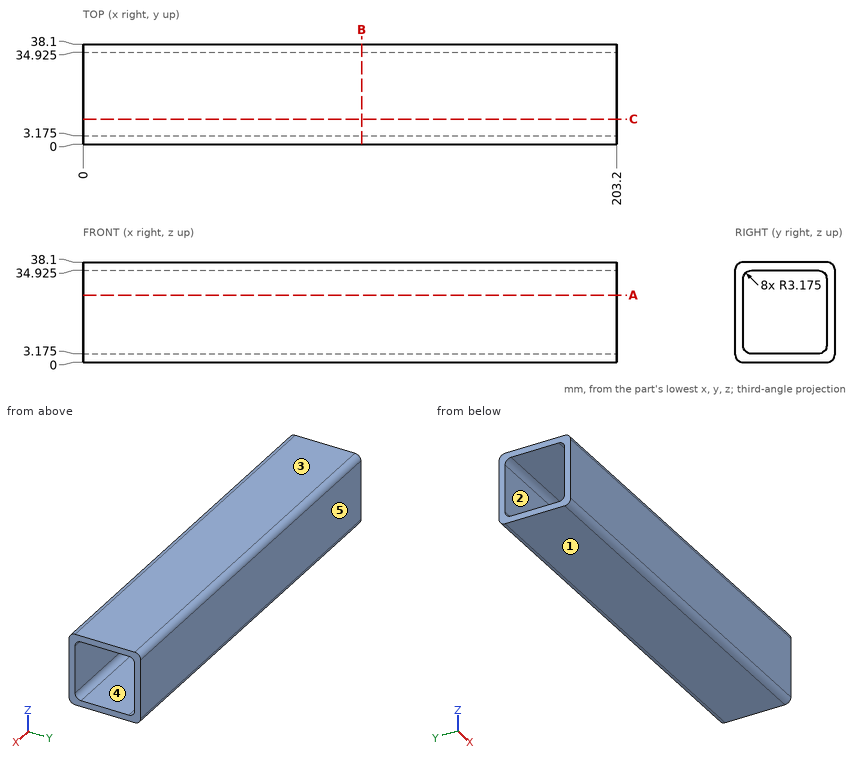
Source: three-view drawing plus pictorial views. Frame: mm from the lowest corner of the part. A direction names the side the tool comes from. Round coordinates to 2 decimals unless told otherwise and drop trailing zeros. Write each loop counter-clockwise with the first axis right and the second up, starting at its lowest first coordinate (ties: lowest second). Pieces come first, ordered by that corner, then holes. Notation, with made-up numbers: M 69,19.5 L 99,19.5 A15 ccw 99,42.5 Z; hole C -27,22.25 d6. An arc over 180 degrees is marked long. Write item = value, one per line.
Item 1: Material intervals for line 1 along Y through (x, z) = (79, 18) (3 decimals); line 2 along Y through (x, z) = (167, 5), sorted ascending. Write a range as [from, to].
Findings:
line_1 = [0, 3.175], [34.925, 38.1]
line_2 = [0, 3.48], [34.62, 38.1]
Item 2: Pin query (flat end, axial travel): P1, Ø4, axis at y = 32.5, z = 28, coming from the +X side. Return the tip coordinate at first contact, or that it passes through.
Findings:
P1 = through
Item 3: Section query A-A on z = 25.5. Return loops of the section in (x, y) (3 decimals), then the cut area to 3 significant figures.
Findings:
outline = M 0,0 L 203.2,0 L 203.2,3.175 L 0,3.175 Z; M 0,34.925 L 203.2,34.925 L 203.2,38.1 L 0,38.1 Z
area = 1,290 mm^2
Item 4: Access query for the marked faces 1 and 2. Directions: +Z, -Z, +X, -X, +Y, -Y. A direction counts if a zero-diameter tool reaches every point of the face in a straight line with its end or side. Return the directions, or none.
Findings:
face_1 = -Z, +X, -X, +Y, -Y
face_2 = +X, -X
Item 5: Pull-direction query (Y, two-part tool) for the marked faces 3, 4 and 5; classes: pulls with the +Y half, pulls with the -Y half, needs draft (parallel to the pull), parting line crosses it, or undercut.
Findings:
face_3 = needs draft
face_4 = undercut
face_5 = pulls with the +Y half
Item 6: Section query B-B on x = 106. Return loops of the section in (y, z) (3 decimals).
Findings:
outline = M 0,3.175 A3.175 ccw 3.175,0 L 34.925,0 A3.175 ccw 38.1,3.175 L 38.1,34.925 A3.175 ccw 34.925,38.1 L 3.175,38.1 A3.175 ccw 0,34.925 Z; hole M 3.175,6.35 A3.175 ccw 6.35,3.175 L 31.75,3.175 A3.175 ccw 34.925,6.35 L 34.925,31.75 A3.175 ccw 31.75,34.925 L 6.35,34.925 A3.175 ccw 3.175,31.75 Z
